Geometry check sheet. Reference: the model listing, model coordinates, mm. A direction names the side the tool comes from. Round coordinates to 2 decimals unless told otherwise and drop trailing zeros. Write each loop counter-clockwise with the first axis right and the second up, starting at its lowest first coordinate (ties: lowest second). Pieces come first, ordered by that corner, then holes. Notation, with made-up numbers: M -17.75,60 L 30.25,60 A29 cw 30.25,95 Z; hole C -21.75,-35 d7. An arc over 180 degrees is marked long. One line per item, written item: value. Start each with the question number.
1. Section check C-C (y = -1). Count the separate pieces of the cut face and the enclosed holes in it, and give its area (3 significant figures).
2. Release check for a two-part mould opening along Y. For faces 3 (the flat face through (0, 0, 50)), 4 (the flat face through (-1, 0, 47)), 5 (the cylindrical face through (-0.976, 7.436, 39.367)) record: pulls with the +Y half, pulls with the -Y half, needs draft (parallel to the pull), parting line crosses it, or undercut.
3. Depth check by flat-ended pin: P1, Ø1.5, axis at x = 1.5, z = 34, coming from the +Y side; P2, Ø4, axis at x = 5.5, z = 38.5, coming from the -Y side; P3, Ø3, axis at y = -0.5, z = 47.5, coming from the +X side; P4, Ø6, axis at x = 6, z = 33.5, coming from the +Y side. Enter the tip coordinate at first touch or a pass-through.
4. Scan lines: probe 1 along Z at (x, y) = (0, -4); probe 2 along X at (y, z) = (-4.75, 45); probe 3 along Z at (x, y) = (-1, -4.5). Record each from-to range of solid material in increasing order. Write a range as [from, to].
5. Section check B-B (z = 46.25). Record the boundary of the cut face in (x, y), and give its area (3 significant figures).
6. Section check A-A (x = 0). Record the boundary of the cut face in (y, z), and give its area (3 significant figures).
7. Access from +Z, -Z, +X, -X, +Y, -Y to the whole of each face (thin tool, end or side, straight path). Record for faces 1 (the cylindrical face through (0, -7.5, 45)), 2 (the cylindrical face through (-0.54, -3.7, 42.56)).
from build123d import *

# Parameters (mm, degrees)
F0_R      = 12.5
F1_DEPTH  = 20
F2_R      = 9
F3_DEPTH  = 10
F4_R      = 7.5
F5_DEPTH  = 20
F6_R      = 2
F7_SIZE   = 1
F8_R      = 1
F9_R      = 2.5
F9_R_2    = 2
F10_DEPTH = 25
F11_R     = 3.5
F11_R_2   = 2.5
F12_DEPTH = 50
F13_R     = 34.8132917853
F13_R_2   = 3.5
F13_R_3   = 2.5
F14_DEPTH = 80


with BuildPart() as f1:
    # F0 (on Top) → F1 (new body)
    with BuildSketch(Plane.XY):
        Circle(F0_R)
    extrude(amount=F1_DEPTH)

    # F2 (on face) → F3 (join)
    with BuildSketch(Plane.XY.offset(20)):
        Circle(F2_R)
    extrude(amount=F3_DEPTH)

    # F4 (on face) → F5 (join)
    with BuildSketch(Plane.XY.offset(30)):
        Circle(F4_R)
    extrude(amount=F5_DEPTH)

    # F6
    f6_edges = [f1.edges().sort_by_distance(p)[0] for p in [
        (-12.5, 0, 20),
    ]]
    fillet(f6_edges, radius=F6_R)

    # F7
    f7_edges = [f1.edges().sort_by_distance(p)[0] for p in [
        (-9, 0, 30),
    ]]
    chamfer(f7_edges, length=F7_SIZE)

    # F8
    f8_edges = [f1.edges().sort_by_distance(p)[0] for p in [
        (-7.5, 0, 50),
    ]]
    fillet(f8_edges, radius=F8_R)

    # F9 (on Front) → F10 (cut)
    with BuildSketch(Plane.XZ):
        with Locations((0, 45)):
            Circle(F9_R)
        with Locations((0, 45)):
            Circle(F9_R_2, mode=Mode.SUBTRACT)
    extrude(amount=F10_DEPTH, mode=Mode.SUBTRACT)

    # F11 (on face) → F12 (join)
    with BuildSketch(Plane(origin=(0, 0, 0), x_dir=(1, 0, 0), z_dir=(0, 0, -1))):
        Circle(F11_R)
        Circle(F11_R_2, mode=Mode.SUBTRACT)
    extrude(amount=F12_DEPTH)

    # F13 (on face) → F14 (cut, through all)
    with BuildSketch(Plane(origin=(0, 0, -50), x_dir=(1, 0, 0), z_dir=(0, 0, -1))):
        Circle(F13_R)
        Circle(F13_R_2, mode=Mode.SUBTRACT)
        Circle(F13_R_2)
        Circle(F13_R_3, mode=Mode.SUBTRACT)
        Circle(F13_R_3)
    extrude(amount=-F14_DEPTH, mode=Mode.SUBTRACT)


solid = f1.part
Result sheet:
1. separate pieces: 2
1. enclosed holes: 1
1. area: 290 mm2
2. face 3: needs draft
2. face 4: pulls with the -Y half
2. face 5: parting line crosses it
3. P1: stops at y = 7.46
3. P2: stops at y = -6.63
3. P3: stops at x = 7.5
3. P4: stops at y = 6.87
4. probe 1: z = [30, 42.5], [43, 47], [47.5, 50]
4. probe 2: x = [-5.8, -2.5], [-2, 2], [2.5, 5.8]
4. probe 3: z = [30, 42.71], [43.27, 46.73], [47.29, 50]
5. outline: M -2.17,-7.18 L -2.17,0 L -1.56,0 L -1.56,-7.34 A7.5 ccw 1.56,-7.34 L 1.56,0 L 2.17,0 L 2.17,-7.18 A7.5 ccw long Z
5. area: 168 mm2
6. outline: M -7.5,30 L 7.5,30 L 7.5,49 A1 ccw 6.5,50 L -6.5,50 A1 ccw -7.5,49 L -7.5,47.5 L 0,47.5 L 0,47 L -7.5,47 L -7.5,43 L 0,43 L 0,42.5 L -7.5,42.5 Z
6. area: 292 mm2
7. face 1: +Z, -Z, -Y
7. face 2: -Y
